Work out the finished part from the listing and answer in its coordinate system (mm). Face numbers are marked on the shaded views. A direction names the side the tool comes from. Give positions to 0.01 mm unless a question says otherwise; leave off trailing zeros. Write each loop counter-clockwise with the first axis right and the second up, starting at its lowest first coordinate (ties: lowest second). Pieces come first, ordered by that corner, then holes.
1) Find section D-D (x = -12). Determine the outline of the cut face in (y, z), plus the area to 3 significant figures.
2) Given pin 1 Ø4 at (x, y) = (-102, 82) entering from +Z; pin 2 Ø2 at (x, y) = (0, 82) entering from +Z; pin 3 Ø1.5 at (x, y) = (43.5, 66) entering from +Z, each flat-ended and moving along its own axis, determine where each tip first touches the part or whether it passes through.
3) Find section A-A (y = 66). Determine the outline of the cut face in (x, z).
4) A tool of negligible diameter and unlimited length cuts with its end or side. For the marked faces 1 and 2, from which of +Z, -Z, +X, -X, +Y, -Y can it reach the whole face along a straight path? Write none if from no direction.
5) Straight lines are drawn through the part: probe 1 along Y at (x, z) = (0, 87); probe 2 along X at (y, z) = (82, 86.55); probe 3 along Y at (x, z) = (40.5, 69.5). For each, find the intervals that lie inside material, in ascending order.
6) Determine the mould class of the marked faces 3, 4, 5 and 6 for opening direction X: pulls with the +X half, pulls with the -X half, needs draft (parallel to the pull), parting line crosses it, or undercut.
Solid Edge part; units mm, degrees
sketch "Sketch1" plane through (0, 0, 0) normal (0, 0, 1) x (1, 0, 0)
  line L0 (-110, -90) -> (110, -90)
  line L1 (110, -90) -> (110, 90)
  line L2 (110, 90) -> (-110, 90)
  line L3 (-110, 90) -> (-110, -90)
  circle A0 centre (-86, -66) radius 3.25
  circle A1 centre (-86, 66) radius 3.25
  circle A2 centre (86, -66) radius 3.25
  circle A3 centre (86, 66) radius 3.25
extrude "Protrusion1" add sketch "Sketch1" along normal blind 4
sketch "Sketch2" plane through (0, 0, 4) normal (0, 0, 1) x (1, 0, 0)
  line L0 (-110, -90) -> (110, -90)
  line L1 (110, -90) -> (110, 90)
  line L2 (110, 90) -> (-110, 90)
  line L3 (-110, 90) -> (-110, -90)
  line L4 (-107, -87) -> (107, -87)
  line L5 (107, -87) -> (107, 87)
  line L6 (107, 87) -> (-107, 87)
  line L7 (-107, 87) -> (-107, -87)
extrude "ExtrudedProtrusion_2" add sketch "Sketch2" along normal blind 88
sketch "Sketch3" plane through (0, 0, 4) normal (0, 0, 1) x (1, 0, 0)
  circle A0 centre (-102, -82) radius 7
extrude "ExtrudedProtrusion_3" add sketch "Sketch3" along normal blind 88
sketch "Sketch4" plane through (0, 0, 4) normal (0, 0, 1) x (1, 0, 0)
  circle A0 centre (-102, 82) radius 7
extrude "ExtrudedProtrusion_4" add sketch "Sketch4" along normal blind 88
sketch "Sketch5" plane through (0, 0, 4) normal (0, 0, 1) x (1, 0, 0)
  circle A0 centre (102, -82) radius 7
extrude "ExtrudedProtrusion_5" add sketch "Sketch5" along normal blind 88
sketch "Sketch6" plane through (0, 0, 4) normal (0, 0, 1) x (1, 0, 0)
  circle A0 centre (102, 82) radius 7
extrude "ExtrudedProtrusion_6" add sketch "Sketch6" along normal blind 88
sketch "Sketch7" plane through (0, 0, 4) normal (0, 0, 1) x (1, 0, 0)
  circle A0 centre (0, -82) radius 7
extrude "ExtrudedProtrusion_7" add sketch "Sketch7" along normal blind 88
sketch "Sketch8" plane through (0, 0, 4) normal (0, 0, 1) x (1, 0, 0)
  circle A0 centre (0, 82) radius 7
extrude "ExtrudedProtrusion_8" add sketch "Sketch8" along normal blind 88
sketch "Sketch9" plane through (0, 0, 84) normal (0, 0, 1) x (1, 0, 0)
  circle A0 centre (-102, -82) radius 1.7
  circle A1 centre (-102, 82) radius 1.7
  circle A2 centre (102, -82) radius 1.7
  circle A3 centre (102, 82) radius 1.7
  circle A4 centre (0, -82) radius 1.7
  circle A5 centre (0, 82) radius 1.7
extrude "ExtrudedCutout_1" cut sketch "Sketch9" along normal blind 8
sketch "Sketch10" plane through (0, 0, 89.3) normal (0, 0, 1) x (1, 0, 0)
  line L0 (-98.6514, -82) -> (-100.3257, -79.1)
  line L1 (-100.3257, -79.1) -> (-103.6743, -79.1)
  line L2 (-103.6743, -79.1) -> (-105.3486, -82)
  line L3 (-105.3486, -82) -> (-103.6743, -84.9)
  line L4 (-103.6743, -84.9) -> (-100.3257, -84.9)
  line L5 (-100.3257, -84.9) -> (-98.6514, -82)
  line L6 (-98.6514, 82) -> (-100.3257, 84.9)
  line L7 (-100.3257, 84.9) -> (-103.6743, 84.9)
  line L8 (-103.6743, 84.9) -> (-105.3486, 82)
  line L9 (-105.3486, 82) -> (-103.6743, 79.1)
  line L10 (-103.6743, 79.1) -> (-100.3257, 79.1)
  line L11 (-100.3257, 79.1) -> (-98.6514, 82)
  line L12 (105.3486, -82) -> (103.6743, -79.1)
  line L13 (103.6743, -79.1) -> (100.3257, -79.1)
  line L14 (100.3257, -79.1) -> (98.6514, -82)
  line L15 (98.6514, -82) -> (100.3257, -84.9)
  line L16 (100.3257, -84.9) -> (103.6743, -84.9)
  line L17 (103.6743, -84.9) -> (105.3486, -82)
  line L18 (105.3486, 82) -> (103.6743, 84.9)
  line L19 (103.6743, 84.9) -> (100.3257, 84.9)
  line L20 (100.3257, 84.9) -> (98.6514, 82)
  line L21 (98.6514, 82) -> (100.3257, 79.1)
  line L22 (100.3257, 79.1) -> (103.6743, 79.1)
  line L23 (103.6743, 79.1) -> (105.3486, 82)
  line L24 (3.3486, -82) -> (1.6743, -79.1)
  line L25 (1.6743, -79.1) -> (-1.6743, -79.1)
  line L26 (-1.6743, -79.1) -> (-3.3486, -82)
  line L27 (-3.3486, -82) -> (-1.6743, -84.9)
  line L28 (-1.6743, -84.9) -> (1.6743, -84.9)
  line L29 (1.6743, -84.9) -> (3.3486, -82)
  line L30 (3.3486, 82) -> (1.6743, 84.9)
  line L31 (1.6743, 84.9) -> (-1.6743, 84.9)
  line L32 (-1.6743, 84.9) -> (-3.3486, 82)
  line L33 (-3.3486, 82) -> (-1.6743, 79.1)
  line L34 (-1.6743, 79.1) -> (1.6743, 79.1)
  line L35 (1.6743, 79.1) -> (3.3486, 82)
extrude "ExtrudedCutout_2" cut sketch "Sketch10" along normal blind 2.7
sketch "Sketch11" plane through (0, 0, 16) normal (0, 0, 1) x (1, 0, 0)
  line L0 (25, -92) -> (91, -92)
  line L1 (91, -92) -> (91, -84)
  line L2 (91, -84) -> (25, -84)
  line L3 (25, -84) -> (25, -92)
extrude "ExtrudedCutout_3" cut sketch "Sketch11" along normal blind 20
sketch "Sketch12" plane through (0, 0, 0) normal (0, 0, 1) x (1, 0, 0)
  circle A0 centre (17, -43) radius 1.7
  circle A1 centre (63, -43) radius 1.7
  circle A2 centre (17, 18) radius 1.7
  circle A3 centre (63, 18) radius 1.7
extrude "ExtrudedCutout_4" cut sketch "Sketch12" along normal blind 4
sketch "Sketch13" plane through (0, 0, 0) normal (0, 0, 1) x (1, 0, 0)
  circle A0 centre (26, -74) radius 1.7
  circle A1 centre (26, -48) radius 1.7
  circle A2 centre (84, -74) radius 1.7
  circle A3 centre (84, -48) radius 1.7
extrude "ExtrudedCutout_5" cut sketch "Sketch13" along normal blind 4
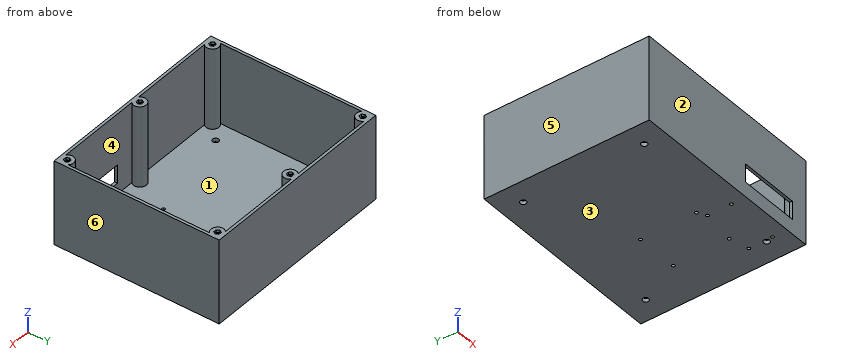
Results:
1. outline: (-90, 0) - (90, 0) - (90, 92) - (87, 92) - (87, 4) - (-87, 4) - (-87, 92) - (-90, 92) - close
1. area: 1,250 mm2
2. pin 1: stops at z = 89.3
2. pin 2: stops at z = 84
2. pin 3: stops at z = 4
3. outline: (-110, 0) - (-89.25, 0) - (-89.25, 4) - (-107, 4) - (-107, 92) - (-110, 92) - close; (-82.75, 0) - (82.75, 0) - (82.75, 4) - (-82.75, 4) - close; (89.25, 0) - (110, 0) - (110, 92) - (107, 92) - (107, 4) - (89.25, 4) - close
4. face 1: +Z
4. face 2: +Z, -Z, +X, -X, -Y
5. probe 1: y = -90 to -83.7, -80.3 to -75, 75 to 80.3, 83.7 to 90
5. probe 2: x = -110 to -103.7, -100.3 to -95, -7 to -1.7, 1.7 to 7, 95 to 100.3, 103.7 to 110
5. probe 3: y = -90 to -87, 87 to 90
6. face 3: needs draft
6. face 4: undercut
6. face 5: pulls with the -X half
6. face 6: pulls with the +X half
